Could you check a few things on this model? Use its own coordinates, in mm. Face numbers are marked on the shaded views. A direction names the side the tool comes from. Coordinates: 2 decimals unless noted, no trailing zeros. Loops run counter-clockwise (first coordinate to the right, second up) from the corner with the lowest first, then second, coordinate; pieces in that order, holes last. Notation, with made-up numbers: M -11,20 L 7,20 A23 ccw 7,38 Z; hole C 24.5,-18.5 d11. An arc over 180 degrees is marked long. Return JSON: item names as keys, results as strings. Group by question number.
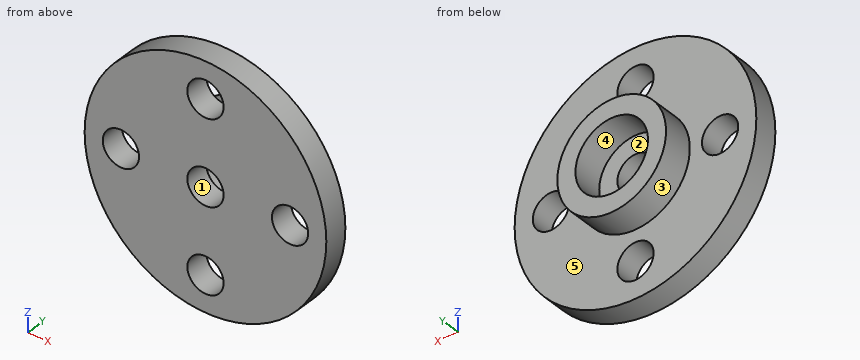
from build123d import *

# Parameters (mm, degrees)
SKETCH1_R           = 10
SKETCH1_R_2         = 1.5
BOSS_EXTRUDE1_DEPTH = 2
SKETCH2_R           = 4.5
SKETCH2_R_2         = 3
BOSS_EXTRUDE2_DEPTH = 2.5


with BuildPart() as part:
    # Sketch1 → Boss-Extrude1 (new body)
    with BuildSketch(Plane(origin=(0, 0, 0), x_dir=(1, 0, 0), z_dir=(0, 1, 0))):
        Circle(SKETCH1_R)
        with Locations((0, -7)):
            Circle(SKETCH1_R_2, mode=Mode.SUBTRACT)
        with Locations((-7, 0)):
            Circle(SKETCH1_R_2, mode=Mode.SUBTRACT)
        with Locations((0, 7)):
            Circle(SKETCH1_R_2, mode=Mode.SUBTRACT)
        with Locations((7, 0)):
            Circle(SKETCH1_R_2, mode=Mode.SUBTRACT)
        Circle(SKETCH1_R_2, mode=Mode.SUBTRACT)
    extrude(amount=BOSS_EXTRUDE1_DEPTH)

    # Sketch2 → Boss-Extrude2 (add)
    with BuildSketch(Plane(origin=(0, 2, 0), x_dir=(1, 0, 0), z_dir=(0, 1, 0))):
        Circle(SKETCH2_R)
        Circle(SKETCH2_R_2, mode=Mode.SUBTRACT)
    extrude(amount=BOSS_EXTRUDE2_DEPTH)


solid = part.part
(1) Will these pins go through, and if not, where does the flat tip stop? P1, Ø1, axis at x = 5.5, y = 1.5, coming from the -Z side; P2, Ø4, axis at x = 0, z = 7, coming from the +Y side.
(2) Imagine slicing it at A-A, the plane x = 0. Write out the boundary of the cut face in (y, z), then the cut area to 3 significant figures.
(3) Imagine slicing it at C-C, the plane z = -7. Write out the boundary of the cut face in (x, y), then the cut area to 3 significant figures.
(4) Imagine slicing it at B-B, the plane y = 1.25. Write out the boundary of the cut face in (x, z).
(5) We'd pull the mould along Z, two halves only. Please class the marked faces 3, 4 and 5: +Z half, -Z half, draft (parallel to the pull), parting line (faces both ways), or undercut.
(6) If I drill on L1, parallel to X at y = 1.3, z = 0; L2, parallel to Y at x = -0.5, z = -2.75, over which ranges is the centre line in solid material (lowest first)? Write a range as [from, to].
(7) Imagine slicing it at D-D, the plane x = -6.25. Write out the boundary of the cut face in (y, z), then the cut area to 3 significant figures.
(8) For the marked faces 1 and 2, which set-ups out of +Z, -Z, +X, -X, +Y, -Y let a thin tool reach every point of the face, with its end or its side?
Checks:
{
 "1": {"P1": "z = -8.66", "P2": "y = 2"},
 "2": {"outline": "M 0,-10 L 2,-10 L 2,-8.5 L 0,-8.5 Z; M 0,-5.5 L 2,-5.5 L 2,-4.5 L 4.5,-4.5 L 4.5,-3 L 2,-3 L 2,-1.5 L 0,-1.5 Z; M 0,1.5 L 2,1.5 L 2,3 L 4.5,3 L 4.5,4.5 L 2,4.5 L 2,5.5 L 0,5.5 Z; M 0,8.5 L 2,8.5 L 2,10 L 0,10 Z", "area": "29.5 mm²"},
 "3": {"outline": "M -7.14,0 L -1.5,0 L -1.5,2 L -7.14,2 Z; M 1.5,0 L 7.14,0 L 7.14,2 L 1.5,2 Z", "area": "22.6 mm²"},
 "4": {"outline": "C 0,0 d20; hole C -7,0 d3; hole C 0,-7 d3; hole C 0,0 d3; hole C 0,7 d3; hole C 7,0 d3"},
 "5": {"face 3": "parting line", "face 4": "undercut", "face 5": "draft"},
 "6": {"L1": "[-10, -8.5], [-5.5, -1.5], [1.5, 5.5], [8.5, 10]", "L2": "[0, 2]"},
 "7": {"outline": "M 0,-7.81 L 2,-7.81 L 2,-1.3 L 0,-1.3 Z; M 0,1.3 L 2,1.3 L 2,7.81 L 0,7.81 Z", "area": "26.0 mm²"},
 "8": {"face 1": "+Y, -Y", "face 2": "+Y"}
}
